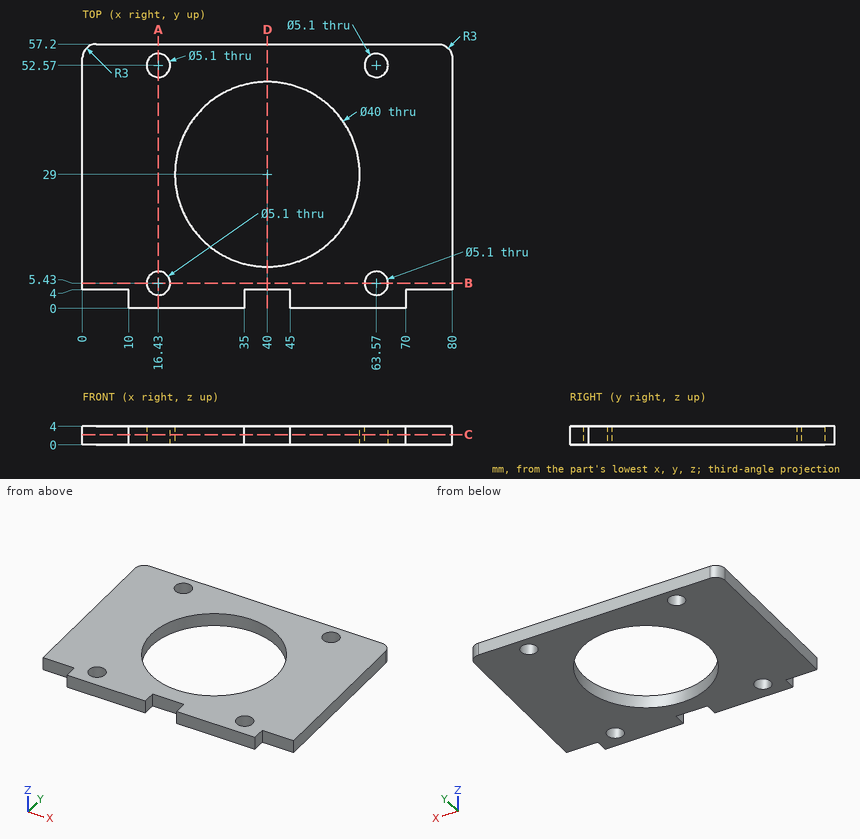
Input: dimensioned drawing with shaded views. Units: mm. Origin: part minimum x, y, z. Coordinates: 2 decimals unless noted, no trailing zeros. Order: outer loops, then holes, each group sorted by start corner. A loop starts at its lowest first (then second) coordinate and runs counter-clockwise, first axis right, second up. Notation, with made-up numbers: (50.5, 18.25) - (75.5, 18.25) arc R24 ccw to (75.5, 53.25) - close; hole circle Ø7 at (-24.5, -15.75). An arc over 180 degrees is marked (long way). Put each result on its own line as item: value.
1. Cut plane A-A on x = 16.43. Return the cut outline in (y, z).
Report:
outline: (0, 0) - (2.88, 0) - (2.88, 4) - (0, 4) - close; (7.98, 0) - (50.02, 0) - (50.02, 4) - (7.98, 4) - close; (55.12, 0) - (57.2, 0) - (57.2, 4) - (55.12, 4) - close
2. Contact query for flat-ended pins moving along their axis: pin 1 Ø1.2 at (y, z) = (2, 1.5) entering from -X; pin 2 Ø1.2 at (x, z) = (73.5, 3) entering from -Y. Output: stop coordinate, or through.
Report:
pin 1: stops at x = 10
pin 2: stops at y = 4
3. Cut plane C-C on z = 2.2. Return the cut outline in (x, y), then the cut area to 3 significant figures.
Report:
outline: (0, 4) - (10, 4) - (10, 0) - (35, 0) - (35, 4) - (45, 4) - (45, 0) - (70, 0) - (70, 4) - (80, 4) - (80, 54.2) arc R3 ccw to (77, 57.2) - (3, 57.2) arc R3 ccw to (0, 54.2) - close; hole circle Ø5.1 at (16.43, 5.43); hole circle Ø5.1 at (16.43, 52.57); hole circle Ø40 at (40, 29); hole circle Ø5.1 at (63.57, 5.43); hole circle Ø5.1 at (63.57, 52.57)
area: 3,110 mm2
4. Cut plane D-D on x = 40. Return the cut outline in (y, z), then the cut area to 3 significant figures.
Report:
outline: (4, 0) - (9, 0) - (9, 4) - (4, 4) - close; (49, 0) - (57.2, 0) - (57.2, 4) - (49, 4) - close
area: 52.8 mm2
5. Line query: line 1 along Y through (x, z) = (16.43, 2.2); line 2 along X through (y, z) = (5.43, 1.2); line 3 along X through (y, z) = (53, 0.4). Output: solid intervals per line, ascending.
Report:
line 1: y = 0 to 2.88, 7.98 to 50.02, 55.12 to 57.2
line 2: x = 0 to 13.88, 18.98 to 61.02, 66.12 to 80
line 3: x = 0 to 13.92, 18.94 to 61.06, 66.08 to 80
6. Cut plane B-B on y = 5.43. Return the cut outline in (x, z).
Report:
outline: (0, 0) - (13.88, 0) - (13.88, 4) - (0, 4) - close; (18.98, 0) - (61.02, 0) - (61.02, 4) - (18.98, 4) - close; (66.12, 0) - (80, 0) - (80, 4) - (66.12, 4) - close
